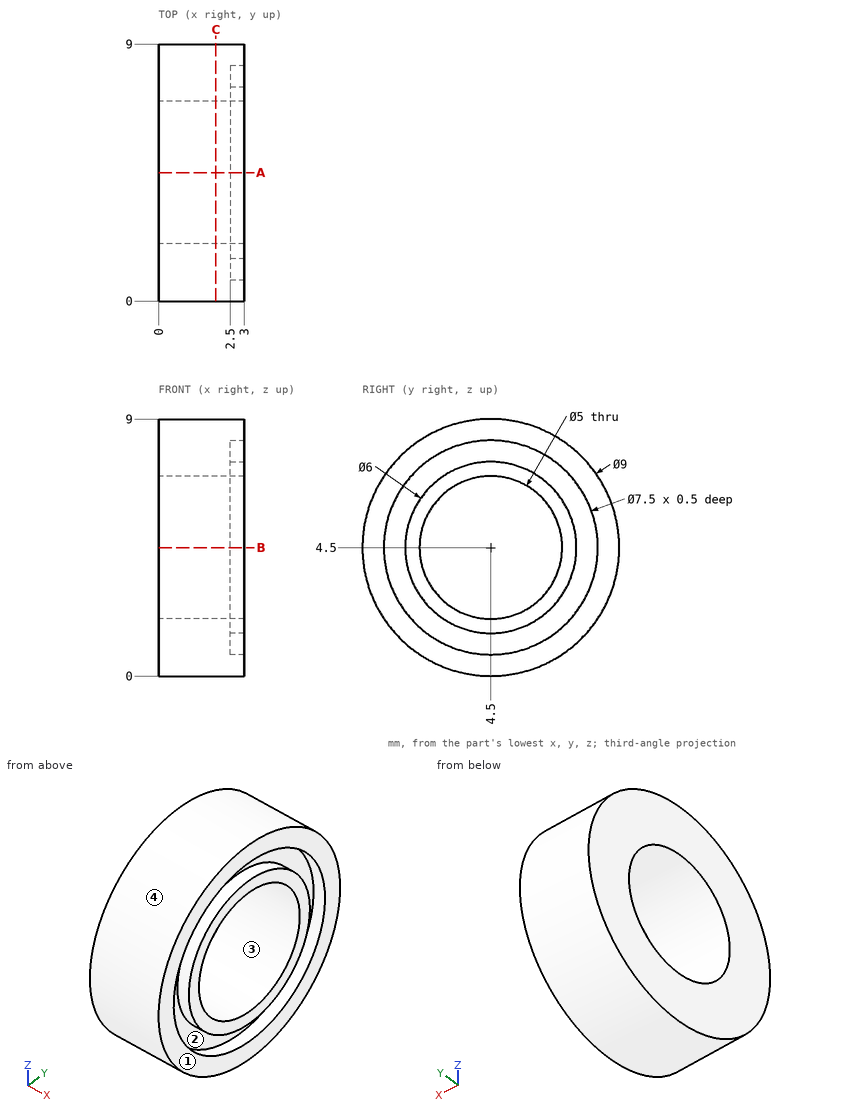
Could you check a few things on this drawing? It's one solid part, dimensions in mm from its lowest x, y, z. Round coordinates to 2 decimals unless told otherwise and drop trailing zeros. Loops run counter-clockwise (first coordinate to the right, second up) from the corner with the lowest first, then second, coordinate; pieces in that order, holes last. Notation, with made-up numbers: M 2,22 L 52,22 A16 ccw 52,27 Z; hole C 11,33 d3. An arc over 180 degrees is marked long. Write item = value, one per line. Start each with the question number.
(1) If we mould it in two halves opening along Y, with no side actions, what happens to the marked faces 1, 2, 3 and 4? For each: released by +Y, released by -Y, zero draft, split by the parting line, or undercut.
(2) Suppose I cut it at C-C on x = 2. Write out the boundary of the cut face in (y, z), plus the area to 3 significant figures.
(3) Suppose I cut it at A-A on y = 4.5. Write out the boundary of the cut face in (x, z).
(4) I'm going to push flat-ended pins straight in: P1, Ø1.5, axis at x = 2.5, z = 5.5, coming from the -Y side; P2, Ø1.5, axis at x = 1.5, y = 3, coming from the -Z side; P3, Ø1.5, axis at x = 2.5, y = 6, coming from the +Z side; P4, Ø2, axis at y = 5.5, z = 3.5, coming from the +X side. Where does each tip first touch, or does it pass through?
(5) I need wall thicknesses on line 1 along Y through (x, z) = (2.9, 4.5); line 2 along Y through (x, z) = (0.75, 4.5); line 3 along X through (y, z) = (8, 3.5). Which ranges of each line are inside material? Lowest first, please.
Answer block:
q1.face_1 = zero draft
q1.face_2 = undercut
q1.face_3 = undercut
q1.face_4 = split by the parting line
q2.outline = C 4.5,4.5 d9; hole C 4.5,4.5 d5
q2.area = 44.0 mm²
q3.outline = M 0,0 L 3,0 L 3,0.75 L 2.5,0.75 L 2.5,1.5 L 3,1.5 L 3,2 L 0,2 Z; M 0,7 L 3,7 L 3,7.5 L 2.5,7.5 L 2.5,8.25 L 3,8.25 L 3,9 L 0,9 Z
q4.P1 = 0.01
q4.P2 = 0.06
q4.P3 = 8.94
q4.P4 = through
q5.line_1 = 0 to 0.75, 1.5 to 2, 7 to 7.5, 8.25 to 9
q5.line_2 = 0 to 2, 7 to 9
q5.line_3 = 0 to 2.5
